Here's how the part is built. I have some questions about the finished solid (model axes, mm). Give positions to 0.01 mm unless a question says otherwise; leave off trailing zeros. Write each loop counter-clockwise with the first axis right and the second up, starting at its lowest first coordinate (ties: lowest second). Pieces come first, ordered by that corner, then holes. Notation, with made-up numbers: (29, 70.5) -> (58, 70.5) arc R21 ccw to (58, 98.5) -> close; hole circle Ø11 at (2.25, -20). An arc over 180 degrees is marked (long way). Use one line per item in the form item = value.
```python
from build123d import *

# Parameters (mm, degrees)
SKETCH2_W           = 71.12
SKETCH2_H           = 6.35
BOSS_EXTRUDE1_DEPTH = 6.35
SKETCH3_R           = 1.143
CUT_EXTRUDE2_DEPTH  = 6.35


with BuildPart() as part:
    # Sketch2 → Boss-Extrude1 (new body)
    with BuildSketch(Plane.XY):
        with Locations((0, 3.175)):
            Rectangle(SKETCH2_W, SKETCH2_H)
    extrude(amount=BOSS_EXTRUDE1_DEPTH)

    # Sketch3 → Cut-Extrude2 (cut)
    with BuildSketch(Plane(origin=(0, 0, 0), x_dir=(1, 0, 0), z_dir=(0, 1, 0))):
        with Locations((-20.6375, -3.175)):
            Circle(SKETCH3_R)
        with Locations((-15.5575, -3.175)):
            Circle(SKETCH3_R)
        with Locations((2.8575, -3.175)):
            Circle(SKETCH3_R)
        with Locations((7.9375, -3.175)):
            Circle(SKETCH3_R)
        with Locations((25.4, -3.175)):
            Circle(SKETCH3_R)
        with Locations((29.21, -3.175)):
            Circle(SKETCH3_R)
    extrude(amount=CUT_EXTRUDE2_DEPTH, mode=Mode.SUBTRACT)


solid = part.part
```
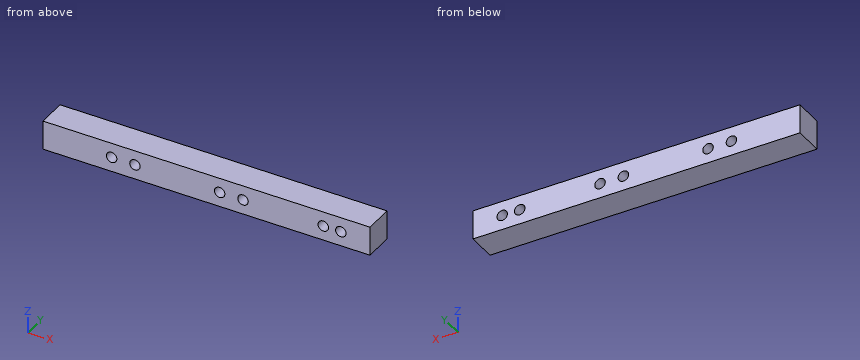
Q1. If I drill on line 1 along Z through (x, y) = (26, 0.5), over which ranges is the centre line in solid material (lowest first)? Write a range as from..to.
Result set:
line_1 = 0..2.2, 4.15..6.35
Q2. I want a section at B-B, the plane y = 1.25. Count the separate pieces of the cut face and the enclosed holes in it, and give its area (3 significant figures).
Result set:
separate_pieces = 1
enclosed_holes = 6
area = 427 mm2
Q3. I want a section at A-A, the plane x = 29.21. Write out the boundary of the cut face in (y, z), and give its area (3 significant figures).
Result set:
outline = (0, 0) -> (6.35, 0) -> (6.35, 2.03) -> (0, 2.03) -> close; (0, 4.32) -> (6.35, 4.32) -> (6.35, 6.35) -> (0, 6.35) -> close
area = 25.8 mm2
